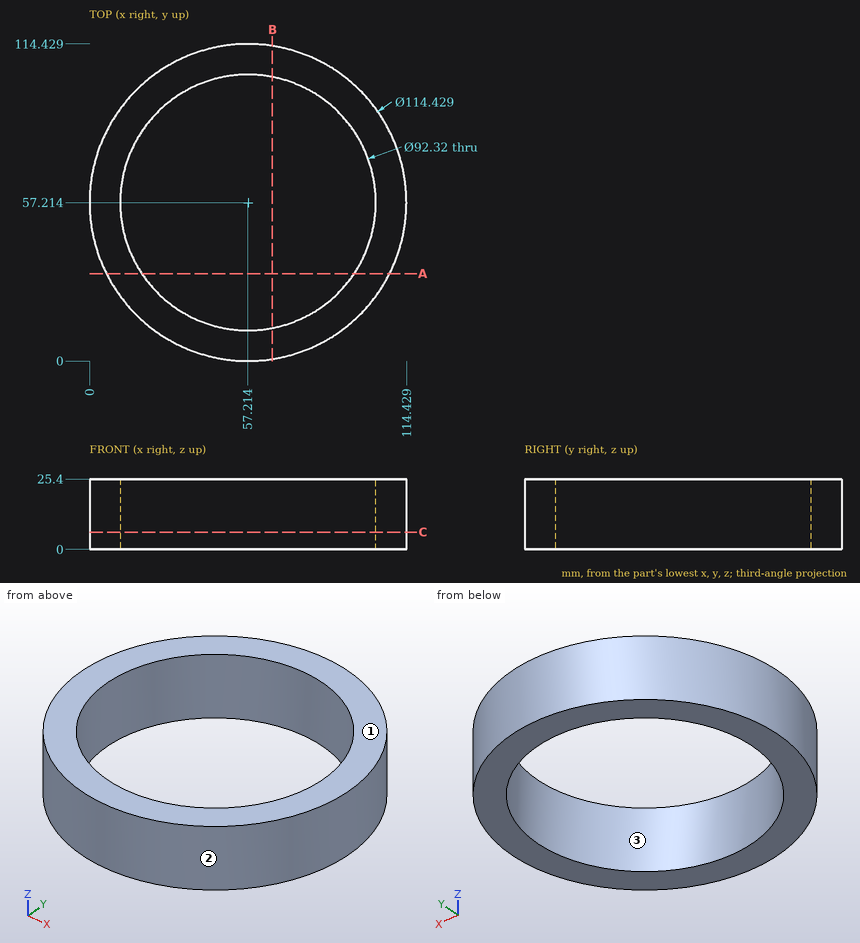
Geometry: see drawing. Coordinates: mm, zero at the bounding-box minimum. Coordinates: 2 decimals unless noted, no trailing zeros. Loops run counter-clockwise (first coordinate to the right, second up) from the corner with the lowest first, then second, coordinate; pieces in that order, holes last. Notation, with made-up numbers: (64, 9) -> (86, 9) arc R24 ccw to (86, 31) -> close; hole circle Ø2 at (44, -32). An arc over 180 degrees is marked (long way). Use a Markdown table: item, result.
1) Material intervals for line 1 along X through (y, z) = (81.5, 21.25); line 2 along Y through (x, z) = (61, 14.5) (1 decimal); line 3 along Y through (x, z) = (20, 4.75) (1 decimal), sorted ascending. Write a range as from..to.
Results found:
| item | result |
|---|---|
| line 1 | x = 5.41..17.96, 96.47..109.02 |
| line 2 | y = 0.1..11.2, 103.2..114.3 |
| line 3 | y = 13.8..29.9, 84.5..100.7 |
2) Cut plane B-B (x = 66). Return the cut outline in (y, z), then the cut area to 3 significant figures.
Results found:
| item | result |
|---|---|
| outline | (0.68, 0) -> (11.9, 0) -> (11.9, 25.4) -> (0.68, 25.4) -> close; (102.53, 0) -> (113.75, 0) -> (113.75, 25.4) -> (102.53, 25.4) -> close |
| area | 570 mm2 |
3) Contact query for flat-ended pins moving along their axis: pin 1 (10 mm diameter, centred on y = 78.5, z = 5, fed in from -X); pin 2 (10 mm diameter, centred on x = 53.5, y = 96, fed in from +Z); pin 3 (10 mm diameter, centred on y = 45, z = 22.5, fed in from -X); pin 4 (12 mm diameter, centred on y = 38, z = 11, fed in from +X). Output: stop coordinate, or through.
Results found:
| item | result |
|---|---|
| pin 1 | stops at x = 2.37 |
| pin 2 | passes through |
| pin 3 | stops at x = 0.46 |
| pin 4 | stops at x = 112.88 |
4) Cut plane C-C (z = 6.25). Return the cut outline in (x, y) (1 decimal), then the cut area to 3 significant figures.
Results found:
| item | result |
|---|---|
| outline | circle Ø114.4 at (57.2, 57.2); hole circle Ø92.3 at (57.2, 57.2) |
| area | 3,590 mm2 |
5) Pull-direction query (X, two-part tool) for the marked faces 1, 2 and 3; classes: released by +X, released by -X, zero draft, split by the parting line, or undercut.
Results found:
| item | result |
|---|---|
| face 1 | zero draft |
| face 2 | split by the parting line |
| face 3 | undercut |
6) Cut plane A-A (y = 31.5). Return the cut outline in (x, z) (1 decimal).
Results found:
| item | result |
|---|---|
| outline | (6.1, 0) -> (18.9, 0) -> (18.9, 25.4) -> (6.1, 25.4) -> close; (95.5, 0) -> (108.3, 0) -> (108.3, 25.4) -> (95.5, 25.4) -> close |
